Verification items for the finished model (mm, model axes). Face numbers are marked on the shaded views. Give positions to 0.01 mm unless a question says otherwise; leave off trailing zeros. Order: outer loops, then holes, each group sorted by start corner. A loop starts at its lowest first (then second) coordinate and runs counter-clockwise, first axis right, second up. Notation, with made-up numbers: (-20.5, 67.25) - (24.5, 67.25) arc R20 ccw to (24.5, 79.25) - close; hole circle Ø1 at (74.25, -26). An arc over 180 degrees is marked (long way). Answer as a JSON object with one key per item and string values.
Solid Edge part; units mm, degrees
sketch "Sketch1" plane through (0, 0, 0) normal (0, 0, 1) x (1, 0, 0)
  line L0 (-21.209, -21.209) -> (21.209, -21.209)
  line L1 (21.209, -21.209) -> (21.209, 21.209)
  line L2 (21.209, 21.209) -> (-21.209, 21.209)
  line L3 (-21.209, 21.209) -> (-21.209, -21.209)
  dimension "D1" = 21.209
  dimension "D2" = 21.209
extrude "Protrusion1" add sketch "Sketch1" along normal blind 6.35
sketch "Sketch2" plane through (0, 0, 6.35) normal (0, 0, 1) x (1, 0, 0)
  circle A0 centre (0, 0) radius 11.049
extrude "MotorMountHole" cut sketch "Sketch2" against normal blind 2.54
sketch "Sketch3" plane through (0, 0, 3.81) normal (0, 0, 1) x (1, 0, 0)
  circle A0 centre (0, 0) radius 6.35
extrude "ShaftHole" cut sketch "Sketch3" against normal blind 25.4
hole "Hole1" at (-15.494, -15.494, 6.35) direction (0, 0, -1) diameter 3 end up to next
hole "Hole2" at (-15.494, 15.494, 6.35) direction (0, 0, -1) diameter 3 end up to next
mirror "Mirror1" about plane through (0, 0, 0) normal (1, 0, 0) of "Hole1", "Hole2"
hole "Hole_5" at (0, 15.494, 6.35) direction (0, 0, -1) diameter 2.459 end up to next thread major 3 thread length 50.8
hole "Hole5" at (0, -15.494, 6.35) direction (0, 0, -1) diameter 2.459 end up to next thread major 3 thread length 50.8
properties material "Aluminum, 6061-T6"
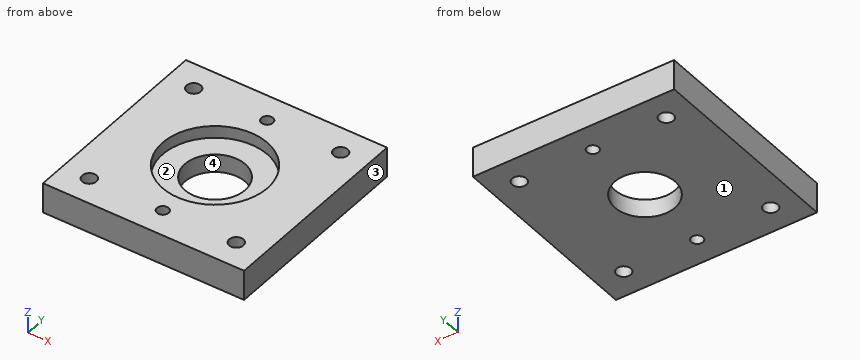
(1) Section check D-D (y = -16). Record the cut outline in (x, z).
Computed values:
{"outline": "(-21.21, 0) - (-16.91, 0) - (-16.91, 6.35) - (-21.21, 6.35) - close; (-14.08, 0) - (-1.12, 0) - (-1.12, 6.35) - (-14.08, 6.35) - close; (1.12, 0) - (14.08, 0) - (14.08, 6.35) - (1.12, 6.35) - close; (16.91, 0) - (21.21, 0) - (21.21, 6.35) - (16.91, 6.35) - close"}
(2) Material ranges on line 1 along X through (y, z) = (-16.5, 3.75); line 2 along Z through (x, y) = (2, 8); line 3 along X through (y, z) = (5.5, 3.25), recorded low to high. Write a range as [from, to].
Computed values:
{"line 1": "x = [-21.21, -16.61], [-14.38, -0.71], [0.71, 14.38], [16.61, 21.21]", "line 2": "z = [0, 3.81]", "line 3": "x = [-21.21, -3.17], [3.17, 21.21]"}
(3) Gauge pin test, flat end, axial feed: pin 1 Ø1.8 at (x, y) = (15.494, -15.494) entering from +Z. Record the tip position at first contact, or that the pin passes through.
Computed values:
{"pin 1": "passes through"}
(4) Section check A-A (y = 0). Record the cut outline in (x, z).
Computed values:
{"outline": "(-21.21, 0) - (-6.35, 0) - (-6.35, 3.81) - (-11.05, 3.81) - (-11.05, 6.35) - (-21.21, 6.35) - close; (6.35, 0) - (21.21, 0) - (21.21, 6.35) - (11.05, 6.35) - (11.05, 3.81) - (6.35, 3.81) - close"}
(5) Release check for a two-part mould opening along X. For the marked faces 1, 2, 3 and 4 record: pulls with the +X half, pulls with the -X half, needs draft (parallel to the pull), parting line crosses it, or undercut.
Computed values:
{"face 1": "needs draft", "face 2": "undercut", "face 3": "pulls with the +X half", "face 4": "undercut"}
(6) Section check C-C (z = 4.75). Record the cut outline in (x, y), then the cut area to 3 significant figures.
Computed values:
{"outline": "(-21.21, -21.21) - (21.21, -21.21) - (21.21, 21.21) - (-21.21, 21.21) - close; hole circle Ø3 at (-15.49, -15.49); hole circle Ø3 at (-15.49, 15.49); hole circle Ø22.1 at (0, 0); hole circle Ø2.46 at (0, -15.49); hole circle Ø2.46 at (0, 15.49); hole circle Ø3 at (15.49, -15.49); hole circle Ø3 at (15.49, 15.49)", "area": "1,380 mm²"}
(7) Section check B-B (x = 0). Record the cut outline in (y, z).
Computed values:
{"outline": "(-21.21, 0) - (-16.72, 0) - (-16.72, 6.35) - (-21.21, 6.35) - close; (-14.26, 0) - (-6.35, 0) - (-6.35, 3.81) - (-11.05, 3.81) - (-11.05, 6.35) - (-14.26, 6.35) - close; (6.35, 0) - (14.26, 0) - (14.26, 6.35) - (11.05, 6.35) - (11.05, 3.81) - (6.35, 3.81) - close; (16.72, 0) - (21.21, 0) - (21.21, 6.35) - (16.72, 6.35) - close"}
